CAD build for the part. Positions are in the model's coordinates, mm. A direction names the side the tool comes from. Round coordinates to 2 decimals unless told otherwise and drop trailing zeros. Loops run counter-clockwise (first coordinate to the right, second up) from the corner with the lowest first, then second, coordinate; pieces in that order, holes last.
from build123d import *

# Parameters (mm, degrees)
SKETCH1_R           = 1.9
BOSS_EXTRUDE1_DEPTH = 1.2
BOSS_EXTRUDE2_DEPTH = 0.6


with BuildPart() as part:
    # Sketch1 → Boss-Extrude1 (new body)
    with BuildSketch(Plane.XY):
        Polygon((-68, 2.514718626), (-65.485281374, 0), (3.485281374, 0), (6, 2.514718626), (6, 42.485281374), (-2.514718626, 51), (-59.485281374, 51), (-68, 42.485281374), align=None)
        with Locations((-0.865721015, 30.964560447)):
            Circle(SKETCH1_R, mode=Mode.SUBTRACT)
        with Locations((-61.134278985, 30.964560447)):
            Circle(SKETCH1_R, mode=Mode.SUBTRACT)
        with Locations((-38.909782256, 8.710806253)):
            Circle(SKETCH1_R, mode=Mode.SUBTRACT)
        with Locations((-23.090217744, 8.710806253)):
            Circle(SKETCH1_R, mode=Mode.SUBTRACT)
        with Locations((-2.804444182, 42.527253566)):
            Circle(SKETCH1_R, mode=Mode.SUBTRACT)
        with Locations((-59.195555818, 42.527253566)):
            Circle(SKETCH1_R, mode=Mode.SUBTRACT)
        with BuildLine():
            Line((3, 27.964560447), (-0.865721015, 27.964560447))
            ThreePointArc((-0.865721015, 27.964560447), (-3.039785544, 28.897329588), (-3.861916537, 31.115598164))
            Line((-3.861916537, 31.115598164), (-5.759945542, 42.01246068))
            ThreePointArc((-5.759945542, 42.01246068), (-5.793298819, 42.268897298), (-5.804444182, 42.527253566))
            Line((-5.804444182, 42.527253566), (-5.804444182, 48))
            Line((-5.804444182, 48), (-54.195555818, 48))
            Line((-54.195555818, 48), (-54.195555818, 42.527253566))
            ThreePointArc((-54.195555818, 42.527253566), (-54.214131423, 42.096659786), (-54.269720219, 41.669265423))
            Line((-54.269720219, 41.669265423), (-56.134278985, 30.964560447))
            ThreePointArc((-56.134278985, 30.964560447), (-57.598745079, 27.429026541), (-61.134278985, 25.964560447))
            Line((-61.134278985, 25.964560447), (-65, 25.964560447))
            Line((-65, 25.964560447), (-65, 3.757359313))
            Line((-65, 3.757359313), (-64.242640687, 3))
            Line((-64.242640687, 3), (-43.909782256, 3))
            Line((-43.909782256, 3), (-43.909782256, 8.710806253))
            ThreePointArc((-43.909782256, 8.710806253), (-42.445316162, 12.246340159), (-38.909782256, 13.710806253))
            Line((-38.909782256, 13.710806253), (-23.090217744, 13.710806253))
            ThreePointArc((-23.090217744, 13.710806253), (-19.554683838, 12.246340159), (-18.090217744, 8.710806253))
            Line((-18.090217744, 8.710806253), (-18.090217744, 3))
            Line((-18.090217744, 3), (2.242640687, 3))
            Line((2.242640687, 3), (3, 3.757359313))
            Line((3, 3.757359313), (3, 27.964560447))
        make_face(mode=Mode.SUBTRACT)
    extrude(amount=BOSS_EXTRUDE1_DEPTH)

    # Sketch2 → Boss-Extrude2 (add)
    with BuildSketch(Plane.XY.offset(1.2)):
        Polygon((-67, 42.071067812), (-67, 2.928932188), (-65.071067812, 1), (3.071067812, 1), (5, 2.928932188), (5, 42.071067812), (-2.928932188, 50), (-59.071067812, 50), align=None)
        Polygon((-66.4, 41.822539674), (-66.4, 3.177460326), (-64.822539674, 1.6), (2.822539674, 1.6), (4.4, 3.177460326), (4.4, 41.822539674), (-3.177460326, 49.4), (-58.822539674, 49.4), align=None, mode=Mode.SUBTRACT)
    extrude(amount=BOSS_EXTRUDE2_DEPTH)


solid = part.part
Item 1: Cut at B-B (x = -11). List the corners of the cut face in (y, z).
Verdict:
outline: (0, 0) - (3, 0) - (3, 1.2) - (1.6, 1.2) - (1.6, 1.8) - (1, 1.8) - (1, 1.2) - (0, 1.2) - close; (48, 0) - (51, 0) - (51, 1.2) - (50, 1.2) - (50, 1.8) - (49.4, 1.8) - (49.4, 1.2) - (48, 1.2) - close
Item 2: Cut at A-A (y = 19.5). List the corners of the cut face in (x, z).
Verdict:
outline: (-68, 0) - (-65, 0) - (-65, 1.2) - (-66.4, 1.2) - (-66.4, 1.8) - (-67, 1.8) - (-67, 1.2) - (-68, 1.2) - close; (3, 0) - (6, 0) - (6, 1.2) - (5, 1.2) - (5, 1.8) - (4.4, 1.8) - (4.4, 1.2) - (3, 1.2) - close
Item 3: Wall check: L1, parallel to X at y = 6, z = 0.3; L2, parallel to X at y = 4.5, z = 1.6; L3, parallel to Y at x = -7.5, z = 1.65. Give the ranges that are in metal, low to high.
Verdict:
L1: x = -68 to -65, -43.91 to -18.09, 3 to 6
L2: x = -67 to -66.4, 4.4 to 5
L3: y = 1 to 1.6, 49.4 to 50
Item 4: Cut at C-C (z = 0.9). State how many separate pieces and enclosed holes the cut face has, plus the area to 3 significant figures.
Verdict:
separate pieces: 1
enclosed holes: 7
area: 1,200 mm2
Item 5: Mould opens along X. For faces 4 (the flat face through (-65.62, 2.4, 1.5)), 5 (the flat face through (-66.05, 1.98, 1.5)), 6 (the flat face through (4.02, 1.95, 1.5)) say: released by +X, released by -X, zero draft, split by the parting line, or undercut.
Verdict:
face 4: undercut
face 5: released by -X
face 6: released by +X
Item 6: Flat gauge pins, fed straight in: P1, Ø2, axis at x = -32, y = 10, coming from the +Z side; P2, Ø0.5, axis at x = -37, z = 1.5, coming from the -Y side; P3, Ø0.6, axis at y = 44.5, z = 1, coming from the +X side. Where does each tip first touch, or does it go through?
Verdict:
P1: stops at z = 1.2
P2: stops at y = 1
P3: stops at x = 4.29
Item 7: 3-axis set-ups, long thin cutter, end or side, ignore diameter. For faces 1 (the flat face through (-62.98, 46.09, 1.5)), 2 (the flat face through (-4.8, 36.5, 0.6)), 3 (the flat face through (3.6, 2.38, 1.5)): which of +Z, -Z, +X, -X, +Y, -Y reach the whole face in a straight line?
Verdict:
face 1: +Z, -X, +Y
face 2: +Z, -Z
face 3: +Z
